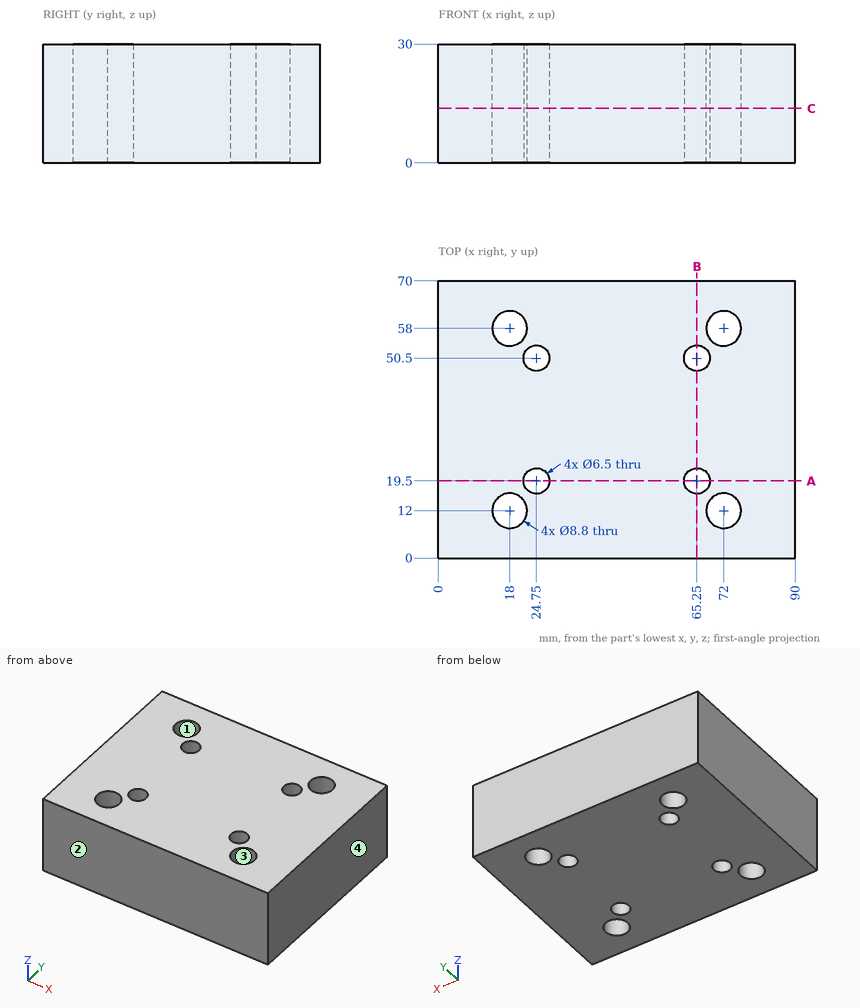
Here's the drawing with two shaded views (mm, measured from the low corner). I have some questions. Round coordinates to 2 decimals unless told otherwise and drop trailing zeros. Write each loop counter-clockwise with the first axis right and the second up, starting at its lowest first coordinate (ties: lowest second). Pieces come first, ordered by that corner, then holes. Notation, with made-up numbers: M -6.5,-16 L 36.5,-16 A24 cw 36.5,10 Z; hole C 65,1 d11. An arc over 180 degrees is marked long. Answer in a Markdown table with one row per item. Add a question column.
Q1. If we mould it in two halves opening along Y, with no side actions, what happens to the marked faces 1, 2, 3 and 4? For each: +Y half, -Y half, draft (parallel to the pull), parting line (faces both ways), or undercut.
Q2. Imagine slicing it at C-C (z = 13.75). Give the number of separate pieces and of enclosed holes in the cut face, then the cut area to 3 significant figures.
Q3. Imagine slicing it at B-B (x = 65.25). Please give me the cut outline in (y, z), then the cut area to 3 significant figures.
Q4. Imagine slicing it at A-A (y = 19.5). Please give me the cut outline in (x, z).
Q5. If I drill on line 1 (Y direction, x = 65.25, z = 15); line 2 (X direction, y = 58, z = 15); line 3 (Y direction, x = 18, z = 15), over which ranges is the centre line in solid material (lowest first)? Write a range as from..to.
Values:
| question | item | result |
|---|---|---|
| 1 | face 1 | undercut |
| 1 | face 2 | -Y half |
| 1 | face 3 | undercut |
| 1 | face 4 | draft |
| 2 | separate pieces | 1 |
| 2 | enclosed holes | 8 |
| 2 | area | 5,920 mm^2 |
| 3 | outline | M 0,0 L 16.25,0 L 16.25,30 L 0,30 Z; M 22.75,0 L 47.25,0 L 47.25,30 L 22.75,30 Z; M 53.75,0 L 70,0 L 70,30 L 53.75,30 Z |
| 3 | area | 1,710 mm^2 |
| 4 | outline | M 0,0 L 21.5,0 L 21.5,30 L 0,30 Z; M 28,0 L 62,0 L 62,30 L 28,30 Z; M 68.5,0 L 90,0 L 90,30 L 68.5,30 Z |
| 5 | line 1 | 0..16.25, 22.75..47.25, 53.75..70 |
| 5 | line 2 | 0..13.6, 22.4..67.6, 76.4..90 |
| 5 | line 3 | 0..7.6, 16.4..53.6, 62.4..70 |
